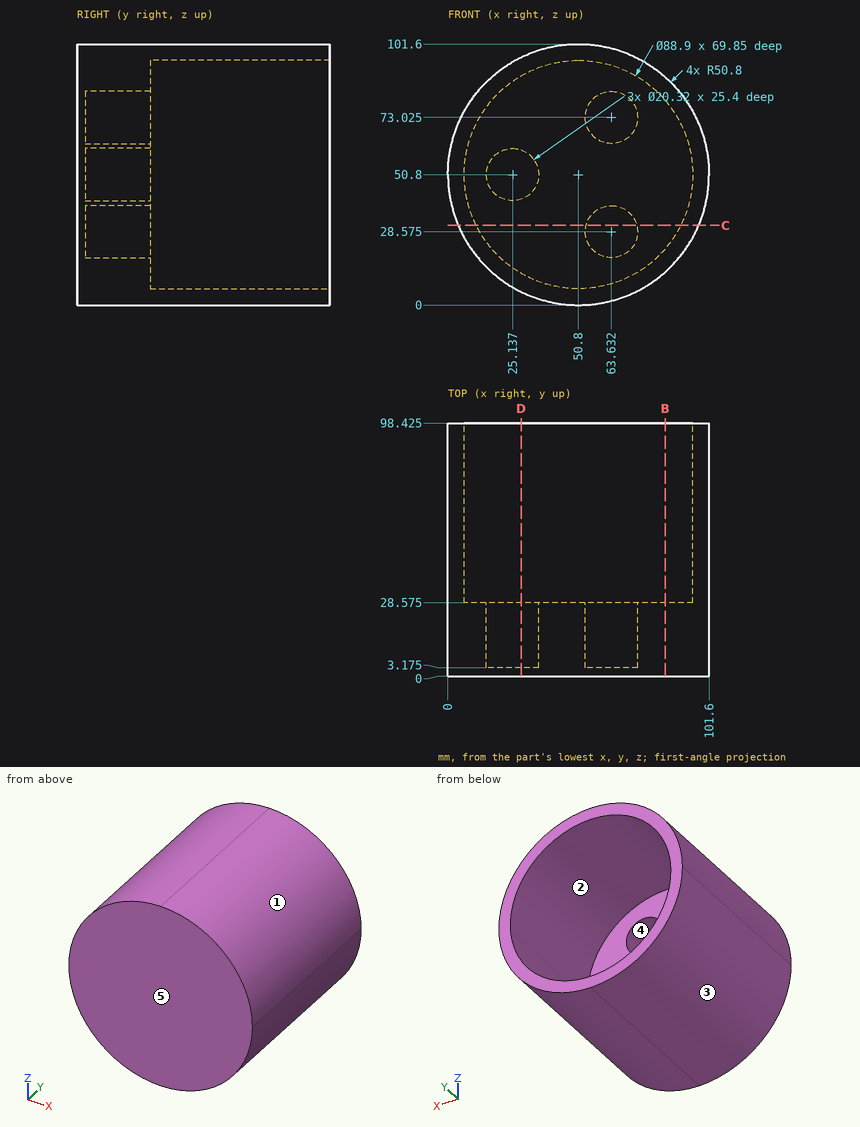
Job drawing, mm, ordinate dimensions from the low corner. One solid piece. A direction names the side the tool comes from. Coordinates: 2 decimals unless noted, no trailing zeros. Loops run counter-clockwise (first coordinate to the right, second up) from the corner with the lowest first, then second, coordinate; pieces in that order, holes last. Notation, with made-up numbers: (64, 68) - (89, 68) arc R7 cw to (89, 75) - close; hole circle Ø2 at (85.25, 71). An arc over 180 degrees is marked (long way). Write item = value, one per line. Start each with the question number.
Q1. Which spindle directions (+Z, -Z, +X, -X, +Y, -Y) get a long thin tool onto all of the face, cutting with end or side? Do the marked faces 1 and 2. Say none if no direction does.
Q2. Pull direction Z, two halves, no side cores. Call the marked faces 3, 4 and 5: pulls with the +Z half, pulls with the -Z half, needs draft (parallel to the pull), parting line crosses it, or undercut.
Q3. Flat gauge pins, fed straight in: pin 1 Ø6 at (y, z) = (50.5, 21) entering from +X (1 decimal); pin 2 Ø5 at (y, z) = (64, 90) entering from +X (1 decimal); pin 3 Ø12 at (y, z) = (37, 10.5) entering from +X. Where does each tip first touch, or does it go through?
Q4. Cut at D-D, the plane x = 28.5. List the corners of the cut face in (y, z) (1 decimal).
Q5. Cut at C-C, the plane z = 31. List the corners of the cut face in (x, y) (1 decimal), then the cut area to 3 significant figures.
Q6. Cut at B-B, the plane x = 84.5. List the corners of the cut face in (y, z) (1 decimal).
Q7. Drill centre lines: L1, parallel to X at y = 83, z = 50; L2, parallel to Z at x = 57, y = 14.5. Where is each one in solid material? Low to high.
Computed:
q1.face_1 = +Z, +X, +Y, -Y
q1.face_2 = +Y
q2.face_3 = pulls with the -Z half
q2.face_4 = undercut
q2.face_5 = needs draft
q3.pin_1 = 94
q3.pin_2 = 85.9
q3.pin_3 = 88.27
q4.outline = (0, 5.2) - (98.4, 5.2) - (98.4, 12.3) - (28.6, 12.3) - (28.6, 41.2) - (3.2, 41.2) - (3.2, 60.4) - (28.6, 60.4) - (28.6, 89.3) - (98.4, 89.3) - (98.4, 96.4) - (0, 96.4) - close
q5.outline = (4, 0) - (97.6, 0) - (97.6, 98.4) - (90.6, 98.4) - (90.6, 28.6) - (73.5, 28.6) - (73.5, 3.2) - (53.8, 3.2) - (53.8, 28.6) - (11, 28.6) - (11, 98.4) - (4, 98.4) - close
q5.area = 3,150 mm²
q6.outline = (0, 12.8) - (98.4, 12.8) - (98.4, 21.8) - (28.6, 21.8) - (28.6, 79.8) - (98.4, 79.8) - (98.4, 88.8) - (0, 88.8) - close
q7.L1 = 0.01 to 6.36, 95.24 to 101.59
q7.L2 = 0.38 to 20.88, 36.27 to 65.33, 80.72 to 101.22
